Geometry: final body of the model. Coordinates: model frame, mm. A direction names the side the tool comes from. Coordinates: 2 decimals unless noted, no trailing zeros. Loops run counter-clockwise (first coordinate to the right, second up) from the corner with the lowest first, then second, coordinate; pieces in that order, holes last. Notation, with made-up numbers: (-16, 31.25) -> (15, 31.25) arc R36 cw to (15, 70.25) -> close; hole circle Ø5 at (58.25, -13). An arc over 180 degrees is marked (long way). One line per item, written item: value. Start each with the question number.
Item 1: Section query A-A on x = -29. Return loops of the section in (y, z).
Item 2: Mould query, pull axis Y, two halves, no side actions, for faces 3 (the flat face through (53.2, 3, 1.6)), 4 (the flat face through (16, -72, 12)). Classes: +Y half, -Y half, draft (parallel to the pull), parting line (faces both ways), or undercut.
Item 3: Ray query, probe 1 along Y at (x, z) = (0, 3.65); probe 2 along Y at (x, z) = (0, 2); probe 3 along Z at (x, y) = (0, -74). Return the intervals inside material, ascending. Write a range as from..to.
Item 4: Set-up query: faces 1 (the flat face through (56.726, 3.045, 1.578)), 2 (the cylindrical face through (-56.998, 0.088, 3.606)). Return all of +Z, -Z, +X, -X, +Y, -Y with unobstructed straight access to the full face (end or side cutting, diameter ignored); none if empty.
Item 5: Section query B-B on y = 17.5. Return loops of the section in (x, z).
Item 6: Contact query for flat-ended pins moving along their axis: pin 1 Ø3 at (y, z) = (41.5, 10.5) entering from +X; pin 2 Ø3.5 at (y, z) = (0, 7) entering from +X; pin 3 Ø2.5 at (x, z) = (0, 2) entering from +Y; pin 4 Ø10 at (x, y) = (-32.5, 49) entering from +Z. Output: stop coordinate, or through.
Item 7: Section query C-C on x = -49.5. Return loops of the section in (y, z).
from build123d import *

# Parameters (mm, degrees)
SKETCH1_R               = 75
SKETCH1_R_2             = 40
BOSS_EXTRUDE1_DEPTH     = 4
SKETCH2_R               = 75
SKETCH2_R_2             = 73
BOSS_EXTRUDE2_DEPTH     = 8
CUT_EXTRUDE1_REACH      = 108.743
CUT_EXTRUDE1_END_RADIUS = 75
SKETCH3_R               = 1.5
CIRPATTERN1_COUNT       = 4
F_4_0MM_DOWEL_HOLE1_D   = 4
CUT_EXTRUDE2_DEPTH      = 3.2


with BuildPart() as part:
    # Sketch1 → Boss-Extrude1 (new body)
    with BuildSketch(Plane.XY):
        Circle(SKETCH1_R)
        Circle(SKETCH1_R_2, mode=Mode.SUBTRACT)
    extrude(amount=BOSS_EXTRUDE1_DEPTH)

    # Sketch2 → Boss-Extrude2 (add)
    with BuildSketch(Plane.XY.offset(4)):
        Circle(SKETCH2_R)
        Circle(SKETCH2_R_2, mode=Mode.SUBTRACT)
    extrude(amount=BOSS_EXTRUDE2_DEPTH)

    # Cut-Extrude1: up to this cylinder (the profile starts inside it)
    cut_extrude1_end = Plane(origin=(0, 0, 7), z_dir=(0, 0, -1)) * Cylinder(CUT_EXTRUDE1_END_RADIUS, 368.486, mode=Mode.PRIVATE)
    # Sketch3 → Cut-Extrude1 (cut, up to the surface)
    with BuildSketch(Plane(origin=(0, 0, 0), x_dir=(1, 0, 0), z_dir=(0, 1, 0)), mode=Mode.PRIVATE) as cut_extrude1_sk1:
        with Locations(Location((0, -7, 0), (0, 0, 270))):
            Circle(SKETCH3_R)
    cut_extrude1_tool1 = extrude(cut_extrude1_sk1.sketch, amount=-CUT_EXTRUDE1_REACH, mode=Mode.PRIVATE) & cut_extrude1_end
    cut_extrude1 = cut_extrude1_tool1.solids().sort_by_distance((0, 0, 7))[0]
    add(cut_extrude1, mode=Mode.SUBTRACT)

    # CirPattern1: Cut-Extrude1 ×4 about axis
    cirpattern1_axis = Axis((0, 0, 4), (0, 0, -1))
    for i in range(1, CIRPATTERN1_COUNT):
        add(cut_extrude1.rotate(cirpattern1_axis, i * 360 / CIRPATTERN1_COUNT), mode=Mode.SUBTRACT)

    # Ø4.0mm Dowel Hole1 (through all)
    with Locations(Plane(origin=(0, 0, 0), x_dir=(-1, 0, 0), z_dir=(0, 0, -1))):
        with Locations((0, 55), (55, 0), (0, -55), (-55, 0)):
            Hole(F_4_0MM_DOWEL_HOLE1_D / 2)

    # Sketch13 → Cut-Extrude2 (cut)
    with BuildSketch(Plane(origin=(0, 0, 0), x_dir=(-1, 0, 0), z_dir=(0, 0, -1))):
        Polygon((4.041451884, 55), (2.020725942, 58.5), (-2.020725942, 58.5), (-4.041451884, 55), (-2.020725942, 51.5), (2.020725942, 51.5), align=None)
        Polygon((55, -4.041451884), (58.5, -2.020725942), (58.5, 2.020725942), (55, 4.041451884), (51.5, 2.020725942), (51.5, -2.020725942), align=None)
        Polygon((-4.041451884, -55), (-2.020725942, -58.5), (2.020725942, -58.5), (4.041451884, -55), (2.020725942, -51.5), (-2.020725942, -51.5), align=None)
        Polygon((-55, 4.041451884), (-58.5, 2.020725942), (-58.5, -2.020725942), (-55, -4.041451884), (-51.5, -2.020725942), (-51.5, 2.020725942), align=None)
    extrude(amount=-CUT_EXTRUDE2_DEPTH, mode=Mode.SUBTRACT)


solid = part.part
Reply:
1. outline: (-69.17, 0) -> (-27.55, 0) -> (-27.55, 4) -> (-66.99, 4) -> (-66.99, 12) -> (-69.17, 12) -> close; (27.55, 0) -> (69.17, 0) -> (69.17, 12) -> (66.99, 12) -> (66.99, 4) -> (27.55, 4) -> close
2. face 3: undercut
2. face 4: draft
3. probe 1: y = -75..-57, -53..-40, 40..53, 57..75
3. probe 2: y = -75..-58.5, -51.5..-40, 40..51.5, 58.5..75
3. probe 3: z = 0..5.5, 8.5..12
4. face 1: -Z
4. face 2: +Z, -Z
5. outline: (-72.93, 0) -> (-35.97, 0) -> (-35.97, 4) -> (-70.87, 4) -> (-70.87, 12) -> (-72.93, 12) -> close; (35.97, 0) -> (72.93, 0) -> (72.93, 12) -> (70.87, 12) -> (70.87, 4) -> (35.97, 4) -> close
6. pin 1: stops at x = 63.44
6. pin 2: stops at x = 75
6. pin 3: stops at y = 75
6. pin 4: stops at z = 4
7. outline: (-56.34, 0) -> (56.34, 0) -> (56.34, 12) -> (53.65, 12) -> (53.65, 4) -> (-53.65, 4) -> (-53.65, 12) -> (-56.34, 12) -> close
